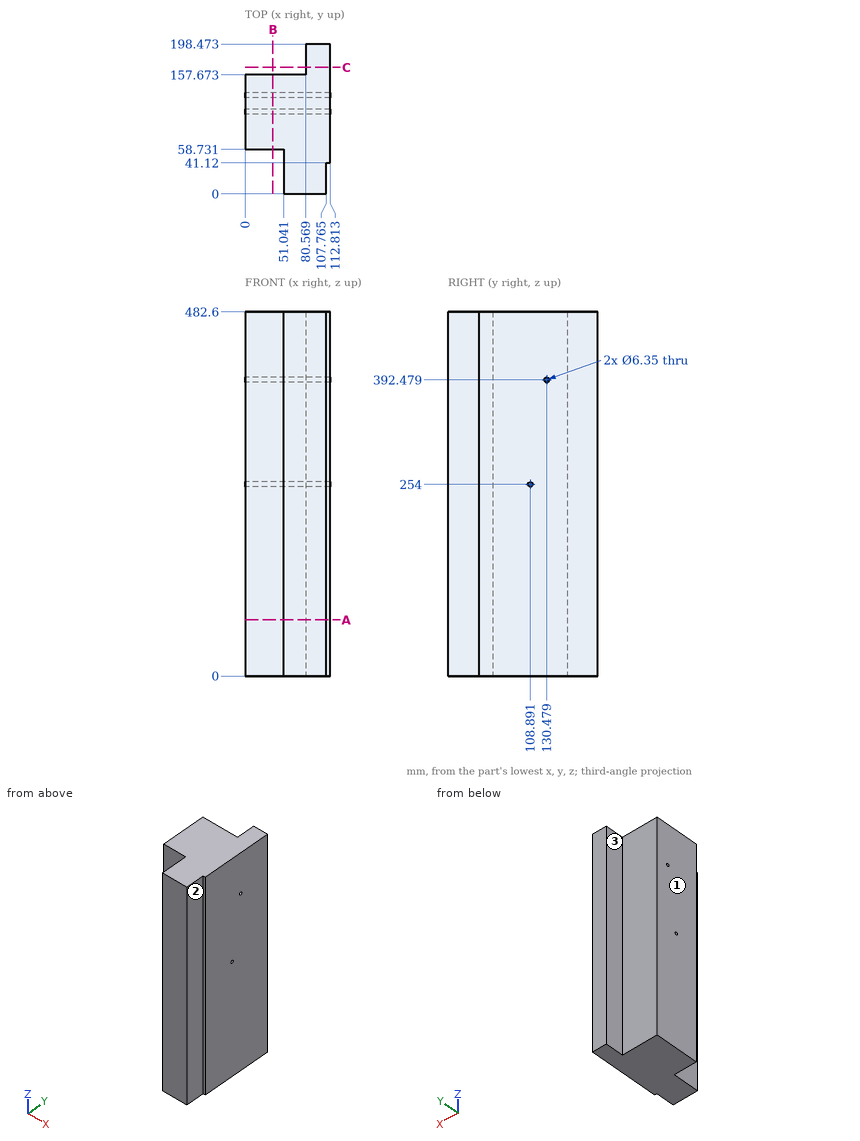
Geometry: see drawing. Coordinates: mm, zero at the bounding-box minimum. A direction names the side the tool comes from. Give positions to 0.01 mm unless a question says otherwise; leave off trailing zeros. Order: outer loops, then holes, each group sorted by start corner. A loop starts at its lowest first (then second) coordinate and runs counter-clockwise, first axis right, second up. Notation, with made-up numbers: M 31.25,31 L 51.25,31 A11 cw 51.25,42 Z; hole C 21.5,15 d6. An arc over 180 degrees is marked long. Answer as CSV lines item,"result". Start each with the question number.
1) Line query: line 1 (Y direction, x = 30.5, z = 254); line 2 (Y direction, x = 30.5, z = 50); line 3 (X direction, y = 45, z = 460.5). Output: solid intervals per line, ascending. Write a range as from..to.
2) Cut plane C-C (y = 167.5). Output: boundary loops of the cut face in (x, z), then the cut area to 3 significant figures.
3) Set-up query: the marked faces 1, 2 and 3. Return all of +Z, -Z, +X, -X, +Y, -Y with unobstructed straight access to the full face (end or side cutting, diameter ignored); none if empty.
4) Cut plane B-B (x = 37). State how many separate pieces and enclosed holes the cut face has, then the cut area to 3 significant figures.
5) First-contact query: P1, Ø12, axis at y = 183.5, z = 330.5, coming from the -X side; P2, Ø2, axis at x = 35, z = 310, coming from the -Y side; P3, Ø8, axis at x = 55.5, z = 208, coming from the -Y side; P4, Ø4, axis at y = 108.89, z = 254, coming from the +X side. Flat tips, straight axial feed; report the tip coordinate or a pass-through.
6) Cut plane A-A (z = 74.5). Output: boundary loops of the cut face in (x, y) (1 decimal), then the cut area to 3 significant figures.
Findings below:
1,line 1,"y = 58.73..105.72, 112.07..157.67"
1,line 2,"y = 58.73..157.67"
1,line 3,"x = 51.04..112.81"
2,outline,"M 80.57,0 L 112.81,0 L 112.81,482.6 L 80.57,482.6 Z"
2,area,"15,600 mm²"
3,face 1,"+Z, -Z, -X, +Y, -Y"
3,face 2,"+Z, -Z, +X, -Y"
3,face 3,"+Z, -Z, -X, +Y"
4,separate pieces,"1"
4,enclosed holes,"2"
4,area,"47,700 mm²"
5,P1,"stops at x = 80.57"
5,P2,"stops at y = 58.73"
5,P3,"stops at y = 0"
5,P4,"passes through"
6,outline,"M 0,58.7 L 51,58.7 L 51,0 L 107.8,0 L 107.8,41.1 L 112.8,41.1 L 112.8,198.5 L 80.6,198.5 L 80.6,157.7 L 0,157.7 Z"
6,area,"15,900 mm²"
